Here's how the part is built. I have some questions about the finished solid (model axes, mm). Round coordinates to 2 decimals unless told otherwise and drop trailing zeros. Write each loop counter-clockwise with the first axis right and the second up, starting at its lowest first coordinate (ties: lowest second). Pieces come first, ordered by that corner, then holes. Notation, with made-up numbers: (40, 1) -> (53, 1) arc R13 ccw to (53, 5) -> close; hole circle Ø2 at (84, -9). An arc over 180 degrees is marked (long way). Answer in a Markdown table with one row per item.
from build123d import *

# Parameters (mm, degrees)
SKETCH1_R           = 105
BOSS_EXTRUDE1_DEPTH = 2
BOSS_EXTRUDE2_START = 2
SKETCH2_R           = 95
BOSS_EXTRUDE2_DEPTH = 45
BOSS_EXTRUDE2_TAPER = 45
CUT_EXTRUDE2_START  = 2
SKETCH3_R           = 95
CUT_EXTRUDE2_DEPTH  = 40
CUT_EXTRUDE2_DRAFT  = -45
CUT_EXTRUDE3_REACH  = 157.753
SKETCH4_R           = 25
CUT_EXTRUDE4_REACH  = 157.753
SKETCH7_R           = 7.5
CIRPATTERN1_COUNT   = 5
CUT_EXTRUDE5_REACH  = 157.753
SKETCH10_R          = 3
CIRPATTERN2_COUNT   = 18
CUT_EXTRUDE7_REACH  = 157.161
SKETCH12_R          = 13.691963716
CIRPATTERN4_COUNT   = 18


with BuildPart() as part:
    # Sketch1 → Boss-Extrude1 (new body)
    with BuildSketch(Plane(origin=(0, 0, 0), x_dir=(1, 0, 0), z_dir=(0, 1, 0))):
        with Locations(Location((0, 0, 0), (0, 0, 270))):
            Circle(SKETCH1_R)
    extrude(amount=BOSS_EXTRUDE1_DEPTH)

    # Sketch2 → Boss-Extrude2 (add)
    with BuildSketch(Plane(origin=(0, 0, 0), x_dir=(1, 0, 0), z_dir=(0, 1, 0)).offset(BOSS_EXTRUDE2_START)):
        Circle(SKETCH2_R)
    extrude(amount=BOSS_EXTRUDE2_DEPTH, taper=BOSS_EXTRUDE2_TAPER)


with BuildPart() as cut_extrude2_tool:
    # Sketch3 → Cut-Extrude2 (with draft: the straight prism first)
    with BuildSketch(Plane.XZ.offset(CUT_EXTRUDE2_START)):
        Circle(SKETCH3_R)
    extrude(amount=-CUT_EXTRUDE2_DEPTH)
    # Cut-Extrude2: the draft: its side faces are tilted about the plane it starts from
    cut_extrude2_sides = [cut_extrude2_tool.faces().sort_by_distance(p)[0] for p in [
        (-95, 18, 0),
    ]]
    draft(cut_extrude2_sides, Plane.XZ.offset(CUT_EXTRUDE2_START), CUT_EXTRUDE2_DRAFT)


with BuildPart() as part_1:
    add(part.part)

    # Cut-Extrude2: cut by cut_extrude2_tool
    add(cut_extrude2_tool.part, mode=Mode.SUBTRACT)

    # Sketch4 → Cut-Extrude3 (cut, up to next)
    with BuildSketch(Plane(origin=(0, 47, 0), x_dir=(1, 0, 0), z_dir=(0, 1, 0)), mode=Mode.PRIVATE) as cut_extrude3_sk1:
        with Locations(Location((0, 0, 0), (0, 0, 270))):
            Circle(SKETCH4_R)
    cut_extrude3_tool1 = extrude(cut_extrude3_sk1.sketch, amount=-CUT_EXTRUDE3_REACH, mode=Mode.PRIVATE) & part_1.part
    add(cut_extrude3_tool1.solids().sort_by_distance((0, 47, 0))[0], mode=Mode.SUBTRACT)

    # Chamfer7: read off the stored shape, not the designer's step
    # Chamfer7 outline → Chamfer7 (revolve, cut)
    with BuildSketch(Plane.XY):
        Polygon((29, 38), (25, 42), (25, 38), align=None)
    revolve(axis=Axis((0, 0, 0), (0, 1, 0)), mode=Mode.SUBTRACT)

    # Sketch7 → Cut-Extrude4 (cut, up to next)
    with BuildSketch(Plane(origin=(0, 47, 0), x_dir=(1, 0, 0), z_dir=(0, 1, 0)), mode=Mode.PRIVATE) as cut_extrude4_sk1:
        with Locations(Location((0, 36.5, 0), (0, 0, 270))):
            Circle(SKETCH7_R)
    cut_extrude4_tool1 = extrude(cut_extrude4_sk1.sketch, amount=-CUT_EXTRUDE4_REACH, mode=Mode.PRIVATE) & part_1.part
    cut_extrude4 = cut_extrude4_tool1.solids().sort_by_distance((0, 47, -36.5))[0]
    add(cut_extrude4, mode=Mode.SUBTRACT)

    # CirPattern1: Cut-Extrude4 ×5 about axis
    cirpattern1_axis = Axis((0, 0, 0), (0, 1, 0))
    for i in range(1, CIRPATTERN1_COUNT):
        add(cut_extrude4.rotate(cirpattern1_axis, i * 360 / CIRPATTERN1_COUNT), mode=Mode.SUBTRACT)

    # Sketch10 → Cut-Extrude5 (cut, up to next)
    with BuildSketch(Plane(origin=(0, 0, 0), x_dir=(1, 0, 0), z_dir=(0, 1, 0)), mode=Mode.PRIVATE) as cut_extrude5_sk1:
        with Locations(Location((0, 100, 0), (0, 0, 270))):
            Circle(SKETCH10_R)
    cut_extrude5_tool1 = extrude(cut_extrude5_sk1.sketch, amount=CUT_EXTRUDE5_REACH, mode=Mode.PRIVATE) & part_1.part
    cut_extrude5 = cut_extrude5_tool1.solids().sort_by_distance((0, 0, -100))[0]
    add(cut_extrude5, mode=Mode.SUBTRACT)

    # CirPattern2: Cut-Extrude5 ×18 about axis
    cirpattern2_axis = Axis((0, 0, 0), (0, 1, 0))
    for i in range(1, CIRPATTERN2_COUNT):
        add(cut_extrude5.rotate(cirpattern2_axis, i * 360 / CIRPATTERN2_COUNT), mode=Mode.SUBTRACT)

    # Cut-Sweep2: sweep along a curve in space
    with BuildLine() as cut_sweep2_path:
        ThreePointArc((0, 38, -55), (38.890872965, 38, -38.890872965), (55, 38, 0))
        ThreePointArc((55, 38, 0), (38.890872965, 38, 38.890872965), (0, 38, 55))
        ThreePointArc((0, 38, 55), (-38.890872965, 38, 38.890872965), (-55, 38, 0))
        ThreePointArc((-55, 38, 0), (-38.890872965, 38, -38.890872965), (0, 38, -55))
    # Sketch9 → Cut-Sweep2 (sweep, cut)
    with BuildSketch(Plane.XY.offset(-13)):
        with BuildLine():
            Line((48.868817725, 37.664960803), (53.784539882, 37.664960803))
            ThreePointArc((53.784539882, 37.664960803), (51.326678803, 39.465568412), (48.868817725, 37.664960803))
        make_face()
    sweep(path=cut_sweep2_path.line, mode=Mode.SUBTRACT)

    # Sketch12 → Cut-Extrude7 (cut, up to next)
    with BuildSketch(Plane(origin=(0, 2, 0), x_dir=(1, 0, 0), z_dir=(0, 1, 0)), mode=Mode.PRIVATE) as cut_extrude7_sk1:
        with Locations((19.25, -109.268280872)):
            Circle(SKETCH12_R)
    cut_extrude7_tool1 = extrude(cut_extrude7_sk1.sketch, amount=-CUT_EXTRUDE7_REACH, mode=Mode.PRIVATE) & part_1.part
    cut_extrude7 = cut_extrude7_tool1.solids().sort_by_distance((19.25, 2, 109.268281))[0]
    add(cut_extrude7, mode=Mode.SUBTRACT)

    # CirPattern4: Cut-Extrude7 ×18 about axis
    cirpattern4_axis = Axis((0, 0, 0), (0, 1, 0))
    for i in range(1, CIRPATTERN4_COUNT):
        add(cut_extrude7.rotate(cirpattern4_axis, i * 360 / CIRPATTERN4_COUNT), mode=Mode.SUBTRACT)


solid = part_1.part
1) We'd pull the mould along Z, two halves only. Please class faces 1 (the face through (10.4, 47, -22.9)), 2 (the face through (16.703, 1.014, -95.816)), 3 (the face through (41.94, 42.56, -13.28)): +Z half, -Z half, draft (parallel to the pull), parting line (faces both ways), or undercut.
Response:
| item | result |
|---|---|
| face 1 | draft |
| face 2 | -Z half |
| face 3 | undercut |
2) I need wall thicknesses on line 1 (Z direction, x = -45.5, y = 44); line 2 (Y direction, x = 47.5, z = 15); line 3 (X direction, y = 1.4, z = -50). Which ranges of each line are inside material? Lowest first, please. Write a range as [from, to].
Response:
| item | result |
|---|---|
| line 1 | z = [-27.18, 27.18] |
| line 2 | y = [38, 47] |
| line 3 | x = [-92.33, -89.6], [-83.6, -76.75], [76.75, 83.6], [89.6, 92.33] |
3) For pin 1 (5 mm diameter, centred on y = 35, z = 55, fed in from -X); pin 2 (3 mm diameter, centred on y = 21.5, z = 27.5, fed in from -X); pin 3 (5.5 mm diameter, centred on x = -64.28, z = -76.6, fed in from -Y); pin 4 (8 mm diameter, centred on x = 34.2, z = 93.97, fed in from -Y), each with a flat end and sliding along its axis, tell me the tip position at first contact or that it passes through.
Response:
| item | result |
|---|---|
| pin 1 | stops at x = -35.13 |
| pin 2 | stops at x = -72.02 |
| pin 3 | passes through |
| pin 4 | stops at y = 0 |
4) I want a section at A-A, the plane y = 11. List the corners of the cut face in (x, z) for me.
Response:
| item | result |
|---|---|
| outline | circle Ø172 at (0, 0); hole circle Ø164 at (0, 0) |
